Verification items for the finished model (mm, model axes). Face numbers are marked on the shaded views. A direction names the side the tool comes from. Give positions to 0.01 mm unless a question says otherwise; leave off trailing zeros. Order: outer loops, then holes, each group sorted by start corner. A loop starts at its lowest first (then second) coordinate and runs counter-clockwise, first axis right, second up.
from build123d import *

# Parameters (mm, degrees)
F1_DEPTH     = 60
F3_DEPTH     = 14
F4_D         = 24.5
F5_T1_DEPTH  = 29.5095436816
F5_T3_DEPTH  = 28.7150489639
F5_T5_DEPTH  = 29.5095436816
F5_T7_DEPTH  = 29.5095436816
F5_T9_DEPTH  = 29.5095436816
F5_T11_DEPTH = 29.5095436816


# Not quite as in the source:
# - a fillet or chamfer that OpenCascade refuses, or shapes differently, is made with other operations: its cross-section is extruded or revolved along the edge and cut away or added


with BuildPart() as f1:
    # F0 (on Front) → F1 (new body)
    with BuildSketch(Plane.XZ):
        with BuildLine():
            Line((-10.5, -22.6881026091), (10.5, -22.6881026091))
            ThreePointArc((10.5, -22.6881026091), (0, 25), (-10.5, -22.6881026091))
        make_face()
    extrude(amount=F1_DEPTH)

    # F2 (on face) → F3 (cut)
    with BuildSketch(Plane(origin=(0, 0, 0), x_dir=(-1, 0, 0), z_dir=(0, 1, 0))):
        with BuildLine():
            ThreePointArc((-24.9341952646, -1.8127069559), (-21.6506350946, -12.5), (-14.0369479057, -20.6872930441))
            Line((-14.0369479057, -20.6872930441), (-24.9341952646, -1.8127069559))
        make_face()
        with BuildLine():
            Line((-24.9341952646, 1.8127069559), (-14.0369479057, 20.6872930441))
            ThreePointArc((-14.0369479057, 20.6872930441), (-21.6506350946, 12.5), (-24.9341952646, 1.8127069559))
        make_face()
        with BuildLine():
            Line((-10.8972473589, 22.5), (10.8972473589, 22.5))
            ThreePointArc((10.8972473589, 22.5), (0, 25), (-10.8972473589, 22.5))
        make_face()
        with BuildLine():
            ThreePointArc((14.0369479057, -20.6872930441), (21.6506350946, -12.5), (24.9341952646, -1.8127069559))
            Line((24.9341952646, -1.8127069559), (14.0369479057, -20.6872930441))
        make_face()
        with BuildLine():
            Line((14.0369479057, 20.6872930441), (24.9341952646, 1.8127069559))
            ThreePointArc((24.9341952646, 1.8127069559), (21.6506350946, 12.5), (14.0369479057, 20.6872930441))
        make_face()
    extrude(amount=-F3_DEPTH, mode=Mode.SUBTRACT)

    # F4 (through all)
    with Locations(Plane(origin=(0, 0, 0), x_dir=(-1, 0, 0), z_dir=(0, 1, 0))):
        with Locations((0, 0)):
            Hole(F4_D / 2)

    # F5: chamfer of 1.5 on 6 edges, made by hand

    # F5_s2 → F5_t1 (cut)
    with BuildSketch(Plane(origin=(-7.3773859204, 0, -12.7780072412), x_dir=(0, 1, 0), z_dir=(0.5, 0, 0.8660254038))):
        Polygon((0, -21), (-1.5, -22.5), (0, -22.5), align=None)
    extrude(amount=F5_T1_DEPTH, mode=Mode.SUBTRACT)

    # F5_s4 → F5_t3 (cut)
    with BuildSketch(Plane.YZ.offset(-14.3575244819)):
        Polygon((-1.5, -22.6881026091), (0, -21.1881026091), (0, -22.6881026091), align=None)
    extrude(amount=F5_T3_DEPTH, mode=Mode.SUBTRACT)

    # F5_s6 → F5_t5 (cut)
    with BuildSketch(Plane(origin=(-7.3773859204, 0, 12.7780072412), x_dir=(0, 1, 0), z_dir=(0.5, 0, -0.8660254038))):
        Polygon((0, -21), (-1.5, -22.5), (0, -22.5), align=None)
    extrude(amount=F5_T5_DEPTH, mode=Mode.SUBTRACT)

    # F5_s8 → F5_t7 (cut)
    with BuildSketch(Plane(origin=(7.3773859204, 0, 12.7780072412), x_dir=(0, 1, 0), z_dir=(-0.5, 0, -0.8660254038))):
        Polygon((0, -21), (-1.5, -22.5), (0, -22.5), align=None)
    extrude(amount=F5_T7_DEPTH, mode=Mode.SUBTRACT)

    # F5_s10 → F5_t9 (cut)
    with BuildSketch(Plane.YZ.offset(-14.7547718408)):
        Polygon((0, 21), (-1.5, 22.5), (0, 22.5), align=None)
    extrude(amount=F5_T9_DEPTH, mode=Mode.SUBTRACT)

    # F5_s12 → F5_t11 (cut)
    with BuildSketch(Plane(origin=(7.3773859204, 0, -12.7780072412), x_dir=(0, 1, 0), z_dir=(-0.5, 0, 0.8660254038))):
        Polygon((0, -21), (-1.5, -22.5), (0, -22.5), align=None)
    extrude(amount=F5_T11_DEPTH, mode=Mode.SUBTRACT)


solid = f1.part
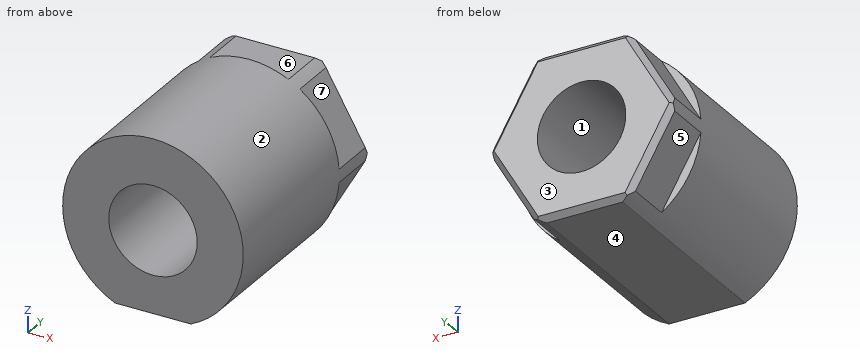
(1) Section check C-C, the plane y = -8.5. Enter the section's corners in (x, z).
Solved:
outline: (-24.93, -1.81) - (-14.04, -20.69) arc R25 ccw to (-10.5, -22.69) - (10.5, -22.69) arc R25 ccw to (14.04, -20.69) - (24.93, -1.81) arc R25 ccw to (24.93, 1.81) - (14.04, 20.69) arc R25 ccw to (10.9, 22.5) - (-10.9, 22.5) arc R25 ccw to (-14.04, 20.69) - (-24.93, 1.81) arc R25 ccw to start; hole circle Ø24.5 at (0, 0)
(2) Section check A-A, the plane x = 0. Enter the section's corners in (y, z), then the cut area to 3 significant figures.
Solved:
outline: (-60, -22.69) - (-1.5, -22.69) - (0, -21.19) - (0, -12.25) - (-60, -12.25) - close; (-60, 12.25) - (0, 12.25) - (0, 21) - (-1.5, 22.5) - (-14, 22.5) - (-14, 25) - (-60, 25) - close
area: 1,350 mm2
(3) Release check for a two-part mould opening along Z. For the marked faces 1, 2 and 3 record: pulls with the +Z half, pulls with the -Z half, needs draft (parallel to the pull), parting line crosses it, or undercut.
Solved:
face 1: undercut
face 2: parting line crosses it
face 3: needs draft
(4) Scan lines: line 1 (Z direction, x = 0, y = -38); line 2 (X direction, y = -3, z = -4); line 3 (Z direction, x = -11, y = -3.5). Record each from-to range of solid material in increasing order.
Solved:
line 1: z = -22.69 to -12.25, 12.25 to 25
line 2: x = -23.67 to -11.58, 11.58 to 23.67
line 3: z = -22.45 to -5.39, 5.39 to 22.45
(5) Section check B-B, the plane z = -6. Enter the section's corners in (x, y).
Solved:
outline: (-24.27, -60) - (-10.68, -60) - (-10.68, 0) - (-20.78, 0) - (-22.52, -1.5) - (-22.52, -14) - (-24.27, -14) - close; (10.68, -60) - (24.27, -60) - (24.27, -14) - (22.52, -14) - (22.52, -1.5) - (20.78, 0) - (10.68, 0) - close
(6) Set-up check for the marked faces 4, 5, 6 and 7: record each of +Z, -Z, +X, -X, +Y, -Y from which the full face is reachable in a straight line by a thin tool's end or side.
Solved:
face 4: -Z, +X, -X, +Y, -Y
face 5: -Z, -X, +Y
face 6: +Z, +X, -X, +Y
face 7: +Z, +X, +Y
(7) Go/stop test with flat-tipped pins: pin 1 (0.8 mm diameter, centred on x = 5, z = 23.5, fed in from +Y); pin 2 (3.5 mm diameter, centred on x = -22, z = 10, fed in from +Y); pin 3 (1.5 mm diameter, centred on y = -40, z = -2, fed in from -X). Record where each tip stops, or that it passes through.
Solved:
pin 1: stops at y = -14
pin 2: stops at y = -1.3
pin 3: stops at x = -24.97
(8) Section check D-D, the plane x = 8. Enter the section's corners in (y, z), then the cut area to 3 significant figures.
Solved:
outline: (-60, -22.69) - (-1.5, -22.69) - (0, -21.19) - (0, -9.28) - (-60, -9.28) - close; (-60, 9.28) - (0, 9.28) - (0, 21) - (-1.5, 22.5) - (-14, 22.5) - (-14, 23.69) - (-60, 23.69) - close
area: 1,650 mm2
